```python
from build123d import *

# Parameters (mm, degrees)
F0_R     = 8.5
F1_DEPTH = 4
F2_R     = 5
F3_DEPTH = 100
F4_W     = 4
F4_H     = 4
F5_DEPTH = 20
F8_R     = 1
F9_DEPTH = 5


with BuildPart() as f1:
    # F0 (on Top) → F1 (new body)
    with BuildSketch(Plane.XY):
        Circle(F0_R)
    extrude(amount=F1_DEPTH)

    # F2 (on Top) → F3 (join)
    with BuildSketch(Plane.XY):
        Circle(F2_R)
    extrude(amount=F3_DEPTH)

    # F4 (on face) → F5 (join)
    with BuildSketch(Plane.XY.offset(100)):
        Rectangle(F4_W, F4_H)
    extrude(amount=F5_DEPTH)

    # F8 (on face) → F9 (join)
    with BuildSketch(Plane(origin=(8.440457, 0.093202, 0), x_dir=(-0.011042, 0.999939, 0), z_dir=(0.999939, 0.011042, 0))):
        with Locations((-0.093208, 2)):
            Circle(F8_R)
    extrude(amount=F9_DEPTH)


solid = f1.part
```
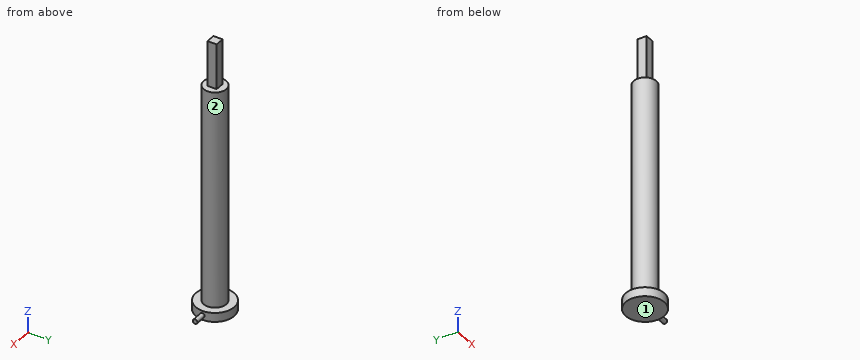
Here's how the part is built. I have some questions about the finished solid (model axes, mm). Face numbers are marked on the shaded views. A direction names the side the tool comes from. Round coordinates to 2 decimals unless told otherwise and drop trailing zeros. Write each loop counter-clockwise with the first axis right and the second up, starting at its lowest first coordinate (ties: lowest second). Pieces come first, ordered by that corner, then holes. Notation, with made-up numbers: M 0.25,46 L 13.25,46 A22 cw 13.25,61 Z; hole C 84.25,42 d11. An arc over 180 degrees is marked long. Answer as CSV lines item,"result". Start each with the question number.
1. Suppose I cut it at A-A on x = 0. Write out the boundary of the cut face in (y, z).
2. I'm going to push flat-ended pins straight in: pin 1 Ø1 at (y, z) = (-6, 22.5) entering from -X; pin 2 Ø1.2 at (x, z) = (-1, 105.5) entering from +Y; pin 3 Ø10 at (y, z) = (5.5, 25.5) entering from +X; pin 4 Ø4.5 at (y, z) = (0, 110.5) entering from -X. Where does each tip first touch, or does it pass through?
3. On a 3-axis mill with a long thin cutter (end or side, diameter ignored), from which of +Z, -Z, +X, -X, +Y, -Y can I reach the whole of each face in a straight line? I mean the marked faces 1 and 2. Say none if no direction works.
4. Suppose I cut it at B-B on z = 82. Write out the boundary of the cut face in (x, y).
5. I need wall thicknesses on probe 1 along Z at (x, y) = (6.25, 4); probe 2 along X at (y, z) = (-1, 52); probe 3 along X at (y, z) = (-2, 35). Which ranges of each line are inside material? Lowest first, please.
6. Suppose I cut it at C-C on y = -7. Write out the boundary of the cut face in (x, z), then the cut area to 3 significant figures.
Check result:
1,outline,"M -8.5,0 L 8.5,0 L 8.5,4 L 5,4 L 5,100 L 2,100 L 2,120 L -2,120 L -2,100 L -5,100 L -5,4 L -8.5,4 Z"
2,pin 1,"passes through"
2,pin 2,"stops at y = 2"
2,pin 3,"stops at x = 4.97"
2,pin 4,"stops at x = -2"
3,face 1,"-Z, +X, -X, +Y, -Y"
3,face 2,"+Z"
4,outline,"C 0,0 d10"
5,probe 1,"z = 0 to 4"
5,probe 2,"x = -4.9 to 4.9"
5,probe 3,"x = -4.58 to 4.58"
6,outline,"M -4.82,0 L 4.82,0 L 4.82,4 L -4.82,4 Z"
6,area,"38.6 mm2"
